from build123d import *

# Parameters (mm, degrees)
BOSS_EXTRUDE1_DEPTH      = 28
BOSS_EXTRUDE1_DEPTH_BACK = 7
SKETCH1_R                = 25
SKETCH1_W                = 50
SKETCH1_H                = 10
SKETCH3_W                = 21.546368229
SKETCH3_H                = 5
BOSS_EXTRUDE2_DEPTH      = 40
CUT_EXTRUDE1_DEPTH       = 238.629693409
CUT_EXTRUDE1_DEPTH_BACK  = 40
SKETCH4_R                = 4
SKETCH5_R                = 4
CUT_EXTRUDE2_DEPTH       = 25
SKETCH6_W                = 15.192054263
SKETCH6_H                = 4
BOSS_EXTRUDE4_DEPTH      = 35
SKETCH7_R                = 4
CUT_EXTRUDE3_DEPTH       = 35
BOSS_EXTRUDE5_DEPTH      = 5
BOSS_EXTRUDE5_DEPTH_BACK = 5
SKETCH8_R                = 4


with BuildPart() as part:
    # Sketch1 → Boss-Extrude1 (new, two sides: drawn at the far end of the back side and taken through both)
    # profile 1 of 3: a face of its own
    with BuildSketch(Plane(origin=(0, 0, 0), x_dir=(0, 0, -1), z_dir=(1, 0, 0)).offset(-BOSS_EXTRUDE1_DEPTH_BACK)):
        Polygon((12.468810267, 220), (12.468810267, 190), (52.468810267, 190), (52.468810267, 205), (52.468810267, 220), align=None)
    # profile 2 of 3: a face of its own
    with BuildSketch(Plane(origin=(0, 0, 0), x_dir=(0, 0, -1), z_dir=(1, 0, 0)).offset(-BOSS_EXTRUDE1_DEPTH_BACK)):
        Polygon((12.468810267, 190), (52.468810267, 190), (30, 136.969027383), (-30, 136.969027383), align=None)
    # profile 3 of 3: a face of its own
    with BuildSketch(Plane(origin=(0, 0, 0), x_dir=(0, 0, -1), z_dir=(1, 0, 0)).offset(-BOSS_EXTRUDE1_DEPTH_BACK)):
        Polygon((-30, 136.969027383), (30, 136.969027383), (30, 106.969027383), (30, 10), (30, -10), (-30, -10), (-30, 10), (-30, 106.969027383), align=None)
        with Locations((0, 106.969027383)):
            Circle(SKETCH1_R, mode=Mode.SUBTRACT)
        Polygon((-25, 20), (-25, 10), (0, 10), (25, 10), (25, 20), align=None, mode=Mode.SUBTRACT)
        Rectangle(SKETCH1_W, SKETCH1_H, mode=Mode.SUBTRACT)
    extrude(amount=BOSS_EXTRUDE1_DEPTH + BOSS_EXTRUDE1_DEPTH_BACK)

    # Sketch3 → Boss-Extrude2 (add)
    with BuildSketch(Plane(origin=(0, 0, -52.468810267), x_dir=(-1, 0, 0), z_dir=(0, 0, -1))):
        with Locations((17.773184115, 192.5)):
            Rectangle(SKETCH3_W, SKETCH3_H)
        with Locations((17.773184115, 217.5)):
            Rectangle(SKETCH3_W, SKETCH3_H)
    extrude(amount=-BOSS_EXTRUDE2_DEPTH)

    # Sketch4 → Cut-Extrude1 (cut, two sides: drawn at the far end of the back side and taken through both)
    with BuildSketch(Plane(origin=(0, 220, 0), x_dir=(1, 0, 0), z_dir=(0, 1, 0)).offset(-CUT_EXTRUDE1_DEPTH_BACK)):
        with Locations(Location((-21.546368229, 32.468810267, 0), (0, 0, 90))):
            Circle(SKETCH4_R)
    extrude(amount=CUT_EXTRUDE1_DEPTH + CUT_EXTRUDE1_DEPTH_BACK, mode=Mode.SUBTRACT)

    # Sketch5 → Cut-Extrude2 (cut)
    with BuildSketch(Plane.XZ.offset(10)):
        with Locations(Location((0, 0, 0), (0, 0, 270))):
            Circle(SKETCH5_R)
    extrude(amount=-CUT_EXTRUDE2_DEPTH, mode=Mode.SUBTRACT)

    # Sketch6 → Boss-Extrude4 (add)
    with BuildSketch(Plane(origin=(0, 0, -30), x_dir=(-1, 0, 0), z_dir=(0, 0, -1))):
        with Locations((-0.596027132, 35.974427815)):
            Rectangle(SKETCH6_W, SKETCH6_H)
        with Locations((-0.596027132, 19.121539986)):
            Rectangle(SKETCH6_W, SKETCH6_H)
    extrude(amount=BOSS_EXTRUDE4_DEPTH)

    # Sketch7 → Cut-Extrude3 (cut)
    with BuildSketch(Plane.XZ.offset(-17.121539986)):
        with Locations(Location((0, -55, 0), (0, 0, 270))):
            Circle(SKETCH7_R)
    extrude(amount=-CUT_EXTRUDE3_DEPTH, mode=Mode.SUBTRACT)

    # Sketch8 → Boss-Extrude5 (add, two sides: drawn at the far end of the back side and taken through both)
    # profile 1 of 2: a face of its own
    with BuildSketch(Plane(origin=(17, 0, 0), x_dir=(0, 0, -1), z_dir=(1, 0, 0)).offset(-BOSS_EXTRUDE5_DEPTH_BACK)):
        with BuildLine():
            Line((-30, 118.060328993), (-30, 64.802844314))
            Line((-30, 64.802844314), (-79.782583008, 83.7497926))
            ThreePointArc((-79.782583008, 83.7497926), (-86.221055725, 93.395743584), (-79.215750464, 102.638254039))
            Line((-79.215750464, 102.638254039), (-30, 118.060328993))
        make_face()
        with Locations((-76.225555525, 93.095784012)):
            Circle(SKETCH8_R, mode=Mode.SUBTRACT)
    # profile 2 of 2: a face of its own
    with BuildSketch(Plane(origin=(17, 0, 0), x_dir=(0, 0, -1), z_dir=(1, 0, 0)).offset(-BOSS_EXTRUDE5_DEPTH_BACK)):
        with BuildLine():
            Line((-30, 47.125470645), (-30, 18.906005285))
            Line((-30, 18.906005285), (-57.203314441, 23.134394747))
            ThreePointArc((-57.203314441, 23.134394747), (-65.667392499, 33.015737965), (-57.203314441, 42.897081183))
            Line((-57.203314441, 42.897081183), (-30, 47.125470645))
        make_face()
        with Locations((-55.667392499, 33.015737965)):
            Circle(SKETCH8_R, mode=Mode.SUBTRACT)
    extrude(amount=BOSS_EXTRUDE5_DEPTH + BOSS_EXTRUDE5_DEPTH_BACK)


solid = part.part
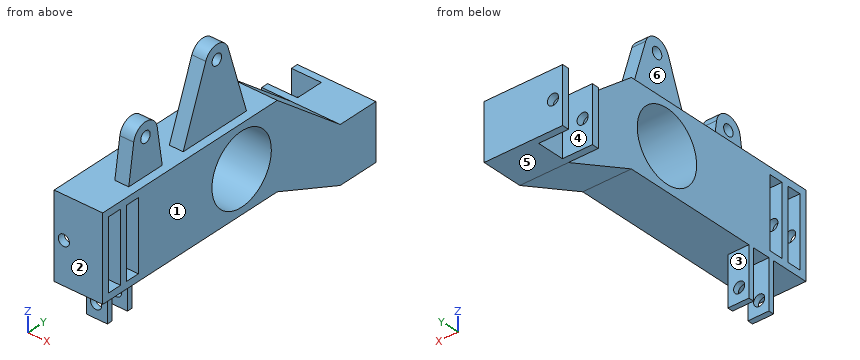
Could you check a few things on this model? Use its own coordinates, in mm. Face numbers are marked on the shaded views. A direction names the side the tool comes from. Give positions to 0.01 mm unless a question says otherwise; leave off trailing zeros. Write each loop counter-clockwise with the first axis right and the second up, starting at its lowest first coordinate (ties: lowest second). Pieces come first, ordered by that corner, then holes. Notation, with made-up numbers: (39.25, 65) -> (43.25, 65) arc R32 ccw to (43.25, 102) -> close; hole circle Ø4 at (68.5, 79). An arc over 180 degrees is marked (long way). Answer as CSV lines item,"result". Start each with the question number.
(1) I'm going to push flat-ended pins straight in: pin 1 Ø6.5 at (x, z) = (-21, -24) entering from -Y; pin 2 Ø5 at (x, y) = (18, 1) entering from +Z; pin 3 Ø4 at (y, z) = (19, 23.5) entering from +X; pin 4 Ø1.5 at (x, y) = (15, 193.5) entering from -Z. Where does each tip first touch, or does it pass through?
(2) If we section it at C-C, the plane x = 0: Give the number of separate pieces and of enclosed holes in the cut face, and give its area (3 significant figures).
(3) Please list where these lines run through material, in increasing order: line 1 (X direction, y = -7, z = 0); line 2 (X direction, y = 20.25, z = -55); line 3 (Y direction, x = 12.5, z = 13).
(4) If we section it at A-A, the plane z = -55: Write out the boundary of the cut face in (x, y).
(5) If we mould it in two halves opening along Y, with no side actions, what happens to the marked faces 1, 2 and 3? For each: +Y half, -Y half, draft (parallel to the pull), parting line (faces both ways), or undercut.
(6) If we section it at D-D, the plane y = 67.5: Write out the boundary of the cut face in (x, z).
(7) Which directions (+Z, -Z, +X, -X, +Y, -Y) give clear straight access to the entire face, cutting with the end or side of a thin tool? Please do the marked faces 4, 5 and 6.
(8) If we section it at B-B, the plane z = 48: Write out the boundary of the cut face in (x, y), and give its area (3 significant figures).
Answer list:
1,pin 1,"y = 190"
1,pin 2,"z = 30"
1,pin 3,"x = 28"
1,pin 4,"z = -52.47"
2,separate pieces,"3"
2,enclosed holes,"1"
2,area,"9,840 mm^2"
3,line 1,"-7 to -4, 4 to 28"
3,line 2,"-7 to -4, 4 to 8.19"
3,line 3,"-10 to -5, 5 to 10, 20 to 85.61, 128.32 to 158.2"
4,outline,"(-7, 17.12) -> (-4, 17.12) -> (-4, 21.12) -> (-7, 21.12) -> close; (-7, 33.97) -> (-4, 33.97) -> (-4, 37.97) -> (-7, 37.97) -> close; (4, 17.12) -> (8.19, 17.12) -> (8.19, 21.12) -> (4, 21.12) -> close; (4, 33.97) -> (8.19, 33.97) -> (8.19, 37.97) -> (4, 37.97) -> close"
5,face 1,"draft"
5,face 2,"-Y half"
5,face 3,"undercut"
6,outline,"(-7, -30) -> (28, -30) -> (28, 30) -> (22, 30) -> (22, 37.09) -> (12, 37.09) -> (12, 30) -> (-7, 30) -> close"
7,face 4,"+Z, -Z, -X"
7,face 5,"-Z, +X, -X, +Y"
7,face 6,"+Z, -X, +Y, -Y"
8,outline,"(12, 21.7) -> (22, 21.7) -> (22, 44.33) -> (12, 44.33) -> close; (12, 71.65) -> (22, 71.65) -> (22, 112.42) -> (12, 112.42) -> close"
8,area,"634 mm^2"
